Read the model definition and answer for the solid it produces. Units are mm, in the model's axes. A direction names the side the tool comes from. Coordinates: 2 decimals unless noted, no trailing zeros. Write each loop counter-clockwise with the first axis right and the second up, starting at its lowest first coordinate (ties: lowest second). Pieces come first, ordered by that corner, then holes. Notation, with made-up numbers: (45, 6) - (63, 6) arc R27 cw to (63, 23) - close; hole circle Ø4 at (-33, -16.5). An arc over 180 degrees is marked (long way). Use a Markdown table: item, result.
from build123d import *

# Parameters (mm, degrees)
BOX002_W                    = 100
BOX002_H                    = 100
BOX002_DEPTH                = 50
COMPOUND002_PLACEMENT_ANGLE = 135
BOX003_W                    = 100
BOX003_H                    = 100
BOX003_DEPTH                = 50
COMPOUND003_PLACEMENT_ANGLE = 225
BOX004_W                    = 100
BOX004_H                    = 100
BOX004_DEPTH                = 50
COMPOUND004_PLACEMENT_ANGLE = 315
BOX001_W                    = 100
BOX001_H                    = 100
BOX001_DEPTH                = 50
COMPOUND001_PLACEMENT_ANGLE = 45
CYLINDER002_R               = 1.25
CYLINDER002_DEPTH           = 50
CYLINDER003_R               = 1.25
CYLINDER003_DEPTH           = 50
CYLINDER004_R               = 1.25
CYLINDER004_DEPTH           = 50
CYLINDER005_R               = 1.25
CYLINDER005_DEPTH           = 50
BOX_W                       = 42.3
BOX_H                       = 42.3
BOX_DEPTH                   = 50
CYLINDER_R                  = 11
CYLINDER_DEPTH              = 2
CYLINDER001_R               = 2.5
CYLINDER001_DEPTH           = 24


with BuildPart() as compound002:
    # Box002 → Box002 (new body)
    with BuildSketch(Plane(origin=(26, -50, 0), x_dir=(1, 0, 0), z_dir=(0, 0, 1))):
        with Locations((50, 50)):
            Rectangle(BOX002_W, BOX002_H)
    extrude(amount=BOX002_DEPTH)


with BuildPart() as compound002_1:
    # Compound002 placement: moved
    add(compound002.part.rotate(Axis((0, 0, 0), (0, 0, 1)), COMPOUND002_PLACEMENT_ANGLE))


with BuildPart() as compound003:
    # Box003 → Box003 (new body)
    with BuildSketch(Plane(origin=(26, -50, 0), x_dir=(1, 0, 0), z_dir=(0, 0, 1))):
        with Locations((50, 50)):
            Rectangle(BOX003_W, BOX003_H)
    extrude(amount=BOX003_DEPTH)


with BuildPart() as compound003_1:
    # Compound003 placement: moved
    add(compound003.part.rotate(Axis((0, 0, 0), (0, 0, 1)), COMPOUND003_PLACEMENT_ANGLE))


with BuildPart() as compound004:
    # Box004 → Box004 (new body)
    with BuildSketch(Plane(origin=(26, -50, 0), x_dir=(1, 0, 0), z_dir=(0, 0, 1))):
        with Locations((50, 50)):
            Rectangle(BOX004_W, BOX004_H)
    extrude(amount=BOX004_DEPTH)


with BuildPart() as compound004_1:
    # Compound004 placement: moved
    add(compound004.part.rotate(Axis((0, 0, 0), (0, 0, 1)), COMPOUND004_PLACEMENT_ANGLE))


with BuildPart() as compound005:
    # Box001 → Box001 (new body)
    with BuildSketch(Plane(origin=(26, -50, 0), x_dir=(1, 0, 0), z_dir=(0, 0, 1))):
        with Locations((50, 50)):
            Rectangle(BOX001_W, BOX001_H)
    extrude(amount=BOX001_DEPTH)


with BuildPart() as compound005_1:
    # Compound001 placement: moved
    add(compound005.part.rotate(Axis((0, 0, 0), (0, 0, 1)), COMPOUND001_PLACEMENT_ANGLE))

    # Compound005: union Compound002, Compound003, Compound004
    add(compound002_1.part)
    add(compound003_1.part)
    add(compound004_1.part)


with BuildPart() as cylinder002:
    # Cylinder002 → Cylinder002 (new body)
    with BuildSketch(Plane(origin=(15.5, 15.5, 0), x_dir=(1, 0, 0), z_dir=(0, 0, 1))):
        Circle(CYLINDER002_R)
    extrude(amount=CYLINDER002_DEPTH)


with BuildPart() as cylinder003:
    # Cylinder003 → Cylinder003 (new body)
    with BuildSketch(Plane(origin=(-15.5, 15.5, 0), x_dir=(1, 0, 0), z_dir=(0, 0, 1))):
        Circle(CYLINDER003_R)
    extrude(amount=CYLINDER003_DEPTH)


with BuildPart() as cylinder004:
    # Cylinder004 → Cylinder004 (new body)
    with BuildSketch(Plane(origin=(15.5, -15.5, 0), x_dir=(1, 0, 0), z_dir=(0, 0, 1))):
        Circle(CYLINDER004_R)
    extrude(amount=CYLINDER004_DEPTH)


with BuildPart() as compound:
    # Cylinder005 → Cylinder005 (new body)
    with BuildSketch(Plane(origin=(-15.5, -15.5, 0), x_dir=(1, 0, 0), z_dir=(0, 0, 1))):
        Circle(CYLINDER005_R)
    extrude(amount=CYLINDER005_DEPTH)

    # Compound: union Cylinder002, Cylinder003, Cylinder004
    add(cylinder002.part)
    add(cylinder003.part)
    add(cylinder004.part)


with BuildPart() as cube:
    # Box → Box (new body)
    with BuildSketch(Plane(origin=(-21.15, -21.15, 0), x_dir=(1, 0, 0), z_dir=(0, 0, 1))):
        with Locations((21.15, 21.15)):
            Rectangle(BOX_W, BOX_H)
    extrude(amount=BOX_DEPTH)


with BuildPart() as fusion:
    # Cylinder → Cylinder (new body)
    with BuildSketch(Plane.XY.offset(-2)):
        Circle(CYLINDER_R)
    extrude(amount=CYLINDER_DEPTH)

    # Fusion: union Cube
    add(cube.part)


with BuildPart() as cut001:
    # Cylinder001 → Cylinder001 (new body)
    with BuildSketch(Plane.XY.offset(-24)):
        Circle(CYLINDER001_R)
    extrude(amount=CYLINDER001_DEPTH)

    # Fusion001: union Fusion
    add(fusion.part)

    # Cut: cut Compound
    add(compound.part, mode=Mode.SUBTRACT)

    # Cut001: cut Compound005
    add(compound005_1.part, mode=Mode.SUBTRACT)


solid = cut001.part
(1) The mould has two halves that part along X. Classify faces 3 (the cylindrical face through (-15.66, -14.26, 24.65)), 4 (the cylindrical face through (15.34, -14.26, 24.65)), 5 (the cylindrical face through (-2.38, -10.74, -1.01)), 6 (the flat face through (21.15, 0, 25)): pulls with the +X half, pulls with the -X half, needs draft (parallel to the pull), parting line crosses it, or undercut.
Report:
| item | result |
|---|---|
| face 3 | undercut |
| face 4 | undercut |
| face 5 | parting line crosses it |
| face 6 | pulls with the +X half |
(2) A cutting plane is placed at D-D, the plane y = 12.5. Write down the section's boundary in (x, z).
Report:
| item | result |
|---|---|
| outline | (-21.15, 0) - (21.15, 0) - (21.15, 50) - (-21.15, 50) - close |
(3) A cutting plane is placed at B-B, the plane x = 0. Write down the section's boundary in (y, z), and give its area (3 significant figures).
Report:
| item | result |
|---|---|
| outline | (-21.15, 0) - (-11, 0) - (-11, -2) - (-2.5, -2) - (-2.5, -24) - (2.5, -24) - (2.5, -2) - (11, -2) - (11, 0) - (21.15, 0) - (21.15, 50) - (-21.15, 50) - close |
| area | 2,270 mm² |
(4) Straight lines are drawn through the part: L1, parallel to Y at x = -15.5, z = 18.5; L2, parallel to Y at x = -15, z = 33; L3, parallel to Z at x = -18, y = 1.5. For each, find the intervals that lie inside material, in ascending order.
Report:
| item | result |
|---|---|
| L1 | y = -21.15 to -16.75, -14.25 to 14.25, 16.75 to 21.15 |
| L2 | y = -21.15 to -16.65, -14.35 to 14.35, 16.65 to 21.15 |
| L3 | z = 0 to 50 |
(5) For faces 1 (the flat face through (0, 0, -24)), 2 (the cylindrical face through (-0.54, -2.44, -13.15)), determine the directions among +Z, -Z, +X, -X, +Y, -Y from which every point of the face is accessible in a straight line to the end or side of a thin tool.
Report:
| item | result |
|---|---|
| face 1 | -Z, +X, -X, +Y, -Y |
| face 2 | -Z |
(6) A cutting plane is placed at A-A, the plane z = 43. Write down the section's boundary in (x, y), and give its area (3 significant figures).
Report:
| item | result |
|---|---|
| outline | (-21.15, -15.62) - (-15.62, -21.15) - (15.62, -21.15) - (21.15, -15.62) - (21.15, 15.62) - (15.62, 21.15) - (-15.62, 21.15) - (-21.15, 15.62) - close; hole circle Ø2.5 at (-15.5, -15.5); hole circle Ø2.5 at (-15.5, 15.5); hole circle Ø2.5 at (15.5, -15.5); hole circle Ø2.5 at (15.5, 15.5) |
| area | 1,710 mm² |
(7) Each of these flat-tipped pins is pushed along its axis until it touches: P1, Ø5, axis at y = -3, z = -16, coming from the +X side; P2, Ø4, axis at x = -15.5, y = -15.5, coming from the -Z side. Where does it stop, or does it pass through?
Report:
| item | result |
|---|---|
| P1 | stops at x = 2.45 |
| P2 | stops at z = 0 |
